For this review, take the finished solid that the model builds, in its own axes (mm). Face numbers are marked on the shaded views. A direction names the side the tool comes from. Coordinates: 2 decimals unless noted, no trailing zeros. Write each loop counter-clockwise with the first axis right and the second up, starting at its lowest first coordinate (ties: lowest second). Pieces come first, ordered by that corner, then holes.
```python
from build123d import *

# Parameters (mm, degrees)
PAD_DEPTH            = 33
SKETCH001_W          = 56
SKETCH001_H          = 86
POCKET_DEPTH         = 100.001
SKETCH003_R          = 3.25
POCKET001_DEPTH      = 95.001
POCKET001_DEPTH_BACK = 100.001
POCKET002_DEPTH      = 95.001


with BuildPart() as part:
    # Sketch002 → Pad (new body, symmetric)
    with BuildSketch(Plane.YZ):
        Polygon((-14.1421356237, 14.1421356237), (91.9238815543, 120.2081528017), (113.1370849898, 120.2081528017), (116.6726188958, 123.7436867076), (120.2081528017, 120.2081528017), (120.2081528017, 113.1370849898), (-7.0710678119, -14.1421356237), (-14.1421356237, -14.1421356237), (-17.6776695297, -10.6066017178), (-14.1421356237, -7.0710678119), align=None)
    extrude(amount=PAD_DEPTH, both=True)

    # Sketch001 (on DatumPlane) → Pocket (cut, through all)
    with BuildSketch(Plane(origin=(0, 0, 0), x_dir=(1, 0, 0), z_dir=(0, -0.7071067812, 0.7071067812))):
        with Locations((0, 48)):
            Rectangle(SKETCH001_W, SKETCH001_H)
    extrude(amount=POCKET_DEPTH, mode=Mode.SUBTRACT)

    # Sketch003 (on DatumPlane) → Pocket001 (cut, two sides)
    with BuildSketch(Plane(origin=(0, 0, 0), x_dir=(1, 0, 0), z_dir=(0, -0.7071067812, 0.7071067812))) as pocket001_sk:
        with Locations((-17.5, 160)):
            Circle(SKETCH003_R)
        with Locations((17.5, 160)):
            Circle(SKETCH003_R)
        with Locations((-17.5, -10)):
            Circle(SKETCH003_R)
        with Locations((17.5, -10)):
            Circle(SKETCH003_R)
    extrude(amount=-POCKET001_DEPTH, mode=Mode.SUBTRACT)
    extrude(pocket001_sk.sketch, amount=POCKET001_DEPTH_BACK, mode=Mode.SUBTRACT)

    # Sketch004 (on DatumPlane) → Pocket002 (cut, through all)
    with BuildSketch(Plane(origin=(0, -3.5355339059, 3.5355339059), x_dir=(1, 0, 0), z_dir=(0, -0.7071067812, 0.7071067812))):
        Polygon((-17.5, 170), (-26.1602540378, 165), (-26.1602540378, 155), (-17.5, 150), (-8.8397459622, 155), (-8.8397459622, 165), align=None)
        Polygon((17.5, 170), (8.8397459622, 165), (8.8397459622, 155), (17.5, 150), (26.1602540378, 155), (26.1602540378, 165), align=None)
        Polygon((17.5, 0), (8.8397459622, -5), (8.8397459622, -15), (17.5, -20), (26.1602540378, -15), (26.1602540378, -5), align=None)
        Polygon((-17.5, 0), (-26.1602540378, -5), (-26.1602540378, -15), (-17.5, -20), (-8.8397459622, -15), (-8.8397459622, -5), align=None)
    extrude(amount=POCKET002_DEPTH, mode=Mode.SUBTRACT)


solid = part.part
```
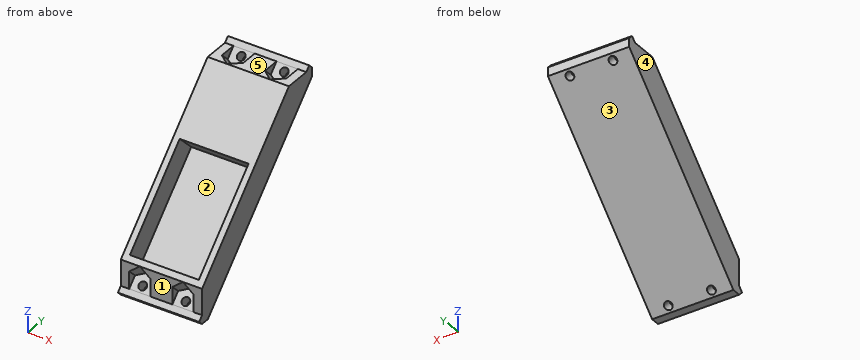
Q1. Add section B-B (x = -10.5). State the section outline as (y, z) points, then the cut area to 3 significant figures.
Ans:
outline: (-17.68, -10.61) - (-14.14, -14.14) - (-7.07, -14.14) - (120.21, 113.14) - (120.21, 120.21) - (116.67, 123.74) - (105.39, 112.46) - (97.64, 120.21) - (91.92, 120.21) - (50.2, 78.49) - (64.35, 64.35) - (3.54, 3.54) - (-10.61, 17.68) - (-14.14, 14.14) - (-14.14, 8.43) - (-6.39, 0.68) - close
area: 2,510 mm2
Q2. For probe 1 along X at (y, z) = (0.5, 13.5); probe 2 along Y at (x, z) = (4, 16.5); probe 3 along Y at (x, z) = (0, 13.5), list the stretches that pass through material, from the lowest coordinate up.
Ans:
probe 1: x = -33 to -28, 28 to 33
probe 2: y = -11.78 to -9.43, 16.5 to 23.57
probe 3: y = -14.14 to -6.43, 13.5 to 20.57
Q3. Add section A-A (y = 58). State the section outline as (x, z) points.
Ans:
outline: (-33, 50.93) - (33, 50.93) - (33, 86.28) - (-33, 86.28) - close; hole (-28, 58) - (28, 58) - (28, 70.69) - (-28, 70.69) - close
Q4. Add section C-C (z = 115). Give the number of separate pieces and of enclosed holes in the cut face, then the cut area to 3 significant figures.
Ans:
separate pieces: 1
enclosed holes: 2
area: 1,870 mm2
Q5. Tool access review of the marked faces 4 and 5: name each direction out of +Z, -Z, +X, -X, +Y, -Y from which nothing blocks a thin tool from reaching the whole face with its end or side.
Ans:
face 4: +Z, -Z, -X, +Y, -Y
face 5: +Z, +X, -X, -Y
Q6. Clearance check with flat-ended pins moving along their axes: pin 1 Ø17 at (x, z) = (21.5, -0.5) entering from -Y; pin 2 Ø8 at (x, y) = (-18.5, 27.5) entering from +Z; pin 3 Ø17 at (x, y) = (2.5, 107.5) entering from +Z. State where each tip first meets the part, or that it passes through.
Ans:
pin 1: stops at y = -16.07
pin 2: stops at z = 31.5
pin 3: stops at z = 123.07
Q7. Draft analysis for pull direction Y (two halves, no side actions). For the marked faces 1, 2 and 3, state which applies: +Y half, -Y half, draft (parallel to the pull), parting line (faces both ways), or undercut.
Ans:
face 1: -Y half
face 2: undercut
face 3: +Y half
Q8. Add section D-D (z = 20). State the section outline as (x, y) points, then the cut area to 3 significant figures.
Ans:
outline: (-33, -8.28) - (-28, -8.28) - (-28, 20) - (28, 20) - (28, -8.28) - (33, -8.28) - (33, 27.07) - (-33, 27.07) - close
area: 750 mm2
